```python
from build123d import *

# Parameters (mm, degrees)
SKETCH2_R           = 2.4
BOSS_EXTRUDE1_DEPTH = 10
SKETCH3_R           = 22
CUT_EXTRUDE1_DEPTH  = 5.03
SKETCH5_R           = 10
CUT_EXTRUDE4_DEPTH  = 5.03


with BuildPart() as part:
    # Sketch2 → Boss-Extrude1 (new body)
    with BuildSketch(Plane(origin=(0, 0, 0), x_dir=(1, 0, 0), z_dir=(0, 1, 0))):
        with BuildLine():
            ThreePointArc((52.570951393, 35.600388644), (52.570951393, 52.570951393), (35.600388644, 52.570951393))
            Line((35.600388644, 52.570951393), (25.836723229, 42.807285978))
            ThreePointArc((25.836723229, 42.807285978), (-0.031141312, 49.999990302), (-25.890026175, 42.775069195))
            Line((-25.890026175, 42.775069195), (-35.685908373, 52.570951393))
            ThreePointArc((-35.685908373, 52.570951393), (-39.559243335, 55.164025054), (-44.128429883, 56.085593835))
            ThreePointArc((-44.128429883, 56.085593835), (-55.180388571, 48.658111405), (-52.570951393, 35.600388644))
            Line((-52.570951393, 35.600388644), (-42.807285978, 25.836723229))
            ThreePointArc((-42.807285978, 25.836723229), (-50, 0), (-42.807285978, -25.836723229))
            Line((-42.807285978, -25.836723229), (-52.570951393, -35.600388644))
            ThreePointArc((-52.570951393, -35.600388644), (-52.570951393, -52.570951393), (-35.600388644, -52.570951393))
            Line((-35.600388644, -52.570951393), (-25.836723229, -42.807285978))
            ThreePointArc((-25.836723229, -42.807285978), (-0.031150905, -49.999990296), (25.783363755, -42.839446232))
            Line((25.783363755, -42.839446232), (27.246595152, -44.30267763))
            ThreePointArc((27.246595152, -44.30267763), (27.683219954, -44.717909015), (28.140137338, -45.110700086))
            Line((28.140137338, -45.110700086), (35.600388644, -52.570951393))
            ThreePointArc((35.600388644, -52.570951393), (52.570951393, -52.570951393), (52.570951393, -35.600388644))
            Line((52.570951393, -35.600388644), (42.807285978, -25.836723229))
            ThreePointArc((42.807285978, -25.836723229), (50, 0), (42.807285978, 25.836723229))
            Line((42.807285978, 25.836723229), (52.570951393, 35.600388644))
        make_face()
        with Locations(Location((-44.085670018, -44.085670018, 0), (0, 0, 270))):
            Circle(SKETCH2_R, mode=Mode.SUBTRACT)
        with BuildLine():
            Line((-18.232233047, -21.767766953), (-28.838834765, -32.374368671))
            ThreePointArc((-28.838834765, -32.374368671), (-32.374368671, -32.374368671), (-32.374368671, -28.838834765))
            Line((-32.374368671, -28.838834765), (-21.767766953, -18.232233047))
            ThreePointArc((-21.767766953, -18.232233047), (-18.232233047, -18.232233047), (-18.232233047, -21.767766953))
        make_face(mode=Mode.SUBTRACT)
        with Locations(Location((44.088384567, -44.088356778, 0), (0, 0, 270))):
            Circle(SKETCH2_R, mode=Mode.SUBTRACT)
        with BuildLine():
            ThreePointArc((32.374368671, -28.838834765), (32.374368671, -32.374368671), (28.838834765, -32.374368671))
            Line((28.838834765, -32.374368671), (18.232233047, -21.767766953))
            ThreePointArc((18.232233047, -21.767766953), (18.232233047, -18.232233047), (21.767766953, -18.232233047))
            Line((21.767766953, -18.232233047), (32.374368671, -28.838834765))
        make_face(mode=Mode.SUBTRACT)
        with BuildLine():
            ThreePointArc((-32.374368671, 28.838834765), (-32.374368671, 32.374368671), (-28.838834765, 32.374368671))
            Line((-28.838834765, 32.374368671), (-18.232233047, 21.767766953))
            ThreePointArc((-18.232233047, 21.767766953), (-18.232233047, 18.232233047), (-21.767766953, 18.232233047))
            Line((-21.767766953, 18.232233047), (-32.374368671, 28.838834765))
        make_face(mode=Mode.SUBTRACT)
        with Locations(Location((-44.085670018, 44.085670018, 0), (0, 0, 270))):
            Circle(SKETCH2_R, mode=Mode.SUBTRACT)
        with BuildLine():
            Line((18.232233047, 21.767766953), (28.838834765, 32.374368671))
            ThreePointArc((28.838834765, 32.374368671), (32.374368671, 32.374368671), (32.374368671, 28.838834765))
            Line((32.374368671, 28.838834765), (21.767766953, 18.232233047))
            ThreePointArc((21.767766953, 18.232233047), (18.232233047, 18.232233047), (18.232233047, 21.767766953))
        make_face(mode=Mode.SUBTRACT)
        with Locations(Location((44.085670018, 44.085670018, 0), (0, 0, 270))):
            Circle(SKETCH2_R, mode=Mode.SUBTRACT)
    extrude(amount=BOSS_EXTRUDE1_DEPTH)

    # Sketch3 → Cut-Extrude1 (cut)
    with BuildSketch(Plane(origin=(0, 0, 0), x_dir=(-1, 0, 0), z_dir=(0, -1, 0))):
        with Locations(Location((0, 0, 0), (0, 0, 90))):
            Circle(SKETCH3_R)
    extrude(amount=-CUT_EXTRUDE1_DEPTH, mode=Mode.SUBTRACT)

    # Sketch5 → Cut-Extrude4 (cut)
    with BuildSketch(Plane(origin=(0, 10, 0), x_dir=(1, 0, 0), z_dir=(0, 1, 0))):
        with Locations(Location((0, 0, 0), (0, 0, 270))):
            Circle(SKETCH5_R)
    extrude(amount=-CUT_EXTRUDE4_DEPTH, mode=Mode.SUBTRACT)


solid = part.part
```
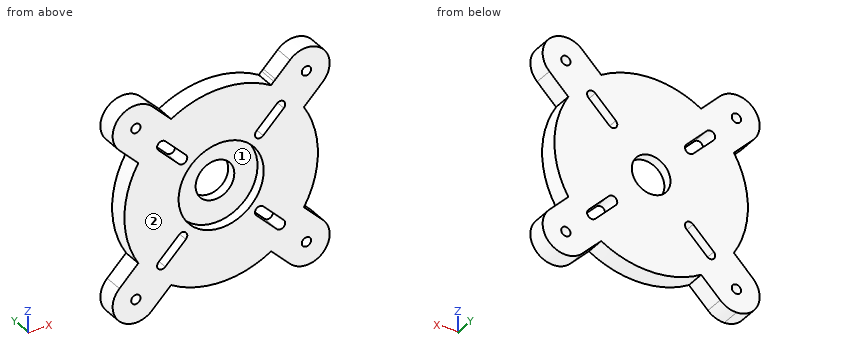
Part model, mm, in its own coordinate system. Face numbers are marked on the shaded views. Round coordinates to 2 decimals unless told otherwise and drop trailing zeros. Loops run counter-clockwise (first coordinate to the right, second up) from the corner with the lowest first, then second, coordinate; pieces in that order, holes last.
1. Slice it at B-B (z = 0). Give the cut face in (x, y).
Solutions:
outline: (-50, 0) - (-22, 0) - (-22, 5.03) - (-10, 5.03) - (-10, 10) - (-50, 10) - close; (10, 5.03) - (22, 5.03) - (22, 0) - (50, 0) - (50, 10) - (10, 10) - close
2. Flat gauge pins, fed straight in: pin 1 (4.5 mm diameter, centred on x = 44.09, z = 44.09, fed in from -Y); pin 2 (6 mm diameter, centred on y = 7, z = -2, fed in from -X); pin 3 (5 mm diameter, centred on x = 10, y = 7.5, fed in from -Z); pin 4 (2 mm diameter, centred on x = 28.5, y = 7, fed in from +Z). Where does each tip first touch, or does it go through?
Solutions:
pin 1: passes through
pin 2: stops at x = -50
pin 3: stops at z = -49.43
pin 4: stops at z = 46.47
3. Slice it at D-D (z = -20). Give the cut face in (x, y).
Solutions:
outline: (-45.83, 0) - (-23.54, 0) - (-23.54, 10) - (-45.83, 10) - close; (-17.5, 0) - (-9.17, 0) - (-9.17, 5.03) - (9.17, 5.03) - (9.17, 0) - (17.5, 0) - (17.5, 10) - (-17.5, 10) - close; (23.54, 0) - (45.83, 0) - (45.83, 10) - (23.54, 10) - close
4. Slice it at A-A (x = 0). Give the cut face in (y, z), and give its area (3 significant figures).
Solutions:
outline: (0, -50) - (10, -50) - (10, -10) - (5.03, -10) - (5.03, -22) - (0, -22) - close; (0, 22) - (5.03, 22) - (5.03, 10) - (10, 10) - (10, 50) - (0, 50) - close
area: 679 mm2
5. Slice it at C-C (x = -23.5). Give the cut face in (y, z), and give its area (3 significant figures).
Solutions:
outline: (0, -44.13) - (10, -44.13) - (10, -27.04) - (0, -27.04) - close; (0, -19.96) - (10, -19.96) - (10, 19.96) - (0, 19.96) - close; (0, 27.04) - (10, 27.04) - (10, 44.13) - (0, 44.13) - close
area: 741 mm2
6. Drill centre lines: line 1 along X through (y, z) = (6, -31.5); line 2 along X through (y, z) = (2.15, 0); line 3 along X through (y, z) = (8.5, -20.5). Where is each one in solid material? Low to high.
Solutions:
line 1: x = -48.47 to -32.94, -27.96 to 27.96, 32.94 to 48.47
line 2: x = -50 to -22, 22 to 50
line 3: x = -45.6 to -24.04, -17.55 to 17.55, 24.04 to 45.6
7. Two-plate mould, pull along Z, no slides. Class the marked faces 1 and 2: pulls with the +Z half, pulls with the -Z half, needs draft (parallel to the pull), parting line crosses it, or undercut.
Solutions:
face 1: undercut
face 2: needs draft
